from build123d import *

# Parameters (mm, degrees)
SKETCH_1_R             = 4
EXTRUDE_1_DEPTH        = 21.25
SKETCH_2_W             = 1
SKETCH_2_H             = 11
CHAMFER_1_SIZE         = 0.5
HOLE_WIZARD_M6_2_D     = 5
HOLE_WIZARD_M6_2_DEPTH = 18
HOLE_WIZARD_M6_2_TIP   = 1.502151548
HOLE_WIZARD_M4_1_D     = 3.3
HOLE_WIZARD_M4_1_DEPTH = 25
HOLE_WIZARD_M4_1_TIP   = 0.991420021
SCALE1_SCALE           = 2


with BuildPart() as part:
    # 草图1 → 凸台-拉伸1 (new, symmetric)
    with BuildSketch(Plane(origin=(0, 0, 0), x_dir=(1, 0, 0), z_dir=(0, 1, 0))):
        with Locations(Location((0, 0, 0), (0, 0, 270))):
            Circle(SKETCH_1_R)
    extrude(amount=EXTRUDE_1_DEPTH, both=True)

    # 草图2 → 旋转1 (revolve)
    with BuildSketch(Plane.XY, mode=Mode.PRIVATE) as revolve_1_sk:
        with Locations((4.5, -15.75)):
            Rectangle(SKETCH_2_W, SKETCH_2_H)
    revolve(revolve_1_sk.sketch.rotate(Axis((0, 21.25, 0), (0, -1, 0)), 270), axis=Axis((0, 21.25, 0), (0, -1, 0)))

    # 倒角1
    chamfer_1_edges = [part.edges().sort_by_distance(p)[0] for p in [
        (0, 21.25, -4),
    ]]
    chamfer(chamfer_1_edges, length=CHAMFER_1_SIZE)

    # M6 螺纹孔2
    with Locations(Plane(origin=(0, -21.25, 0), x_dir=(-1, 0, 0), z_dir=(0, -1, 0))):
        with Locations((0, 0)):
            Hole(HOLE_WIZARD_M6_2_D / 2, depth=HOLE_WIZARD_M6_2_DEPTH)
            with Locations((0, 0, -(HOLE_WIZARD_M6_2_DEPTH + HOLE_WIZARD_M6_2_TIP / 2))):  # 118° drill point
                Cone(0, HOLE_WIZARD_M6_2_D / 2, HOLE_WIZARD_M6_2_TIP, mode=Mode.SUBTRACT)

    # M4 螺纹孔1
    with Locations(Plane(origin=(0, 21.25, 0), x_dir=(1, 0, 0), z_dir=(0, 1, 0))):
        with Locations((0, 0)):
            Hole(HOLE_WIZARD_M4_1_D / 2, depth=HOLE_WIZARD_M4_1_DEPTH)
            with Locations((0, 0, -(HOLE_WIZARD_M4_1_DEPTH + HOLE_WIZARD_M4_1_TIP / 2))):  # 118° drill point
                Cone(0, HOLE_WIZARD_M4_1_D / 2, HOLE_WIZARD_M4_1_TIP, mode=Mode.SUBTRACT)


with BuildPart() as part_1:
    # Scale1: scaled about (0, -1.336200342, 0)
    add(part.part.scale(SCALE1_SCALE).moved(Location((0, 1.336200342, 0))))


solid = part_1.part
Input: part model. Units: mm. Frame: model coordinates. A direction names the side the tool comes from. Coordinates: 2 decimals unless noted, no trailing zeros. Loops run counter-clockwise (first coordinate to the right, second up) from the corner with the lowest first, then second, coordinate; pieces in that order, holes last. Notation, with made-up numbers: (80, -23) -> (134, -23) arc R33 ccw to (134, 8) -> close; hole circle Ø2 at (-32.75, 0.25). An arc over 180 degrees is marked (long way). Write item = value, one per line. Start each with the question number.
Item 1: Material intervals for line 1 (Z direction, x = -6.25, y = -16); line 2 (X direction, y = -35.5, z = 4.5); line 3 (Y direction, x = -8.25, z = 1.25), sorted ascending.
Item 2: Cut plane C-C, the plane y = 37.5. Return loops of the section in (x, z).
Item 3: Cut plane A-A, the plane z = 0. Return loops of the section in (x, y).
Item 4: First-contact query: P1, Ø3, axis at y = 22.5, z = -3, coming from the +X side; P2, Ø1, axis at y = -17, z = -6, coming from the -X side; P3, Ø1.5, axis at x = -2, y = -13, coming from the -Z side. Flat tips, straight axial feed; report the tip coordinate or a pass-through.
Item 5: Reachability of faces 1 (the face through (8.2, -19.164, 0)), 2 (the face through (2.43, 19.51, -2.23)), 3 (the face through (-1.08, -22.91, 4.88)) from +Z, -Z, +X, -X, +Y, -Y: full face, straight path, thin tool, end or side. Return the list, or none.
Item 6: Cut plane B-B, the plane x = 0. Return loops of the section in (y, z).
Item 7: Cut plane D-D, the plane y = -15. Return loops of the section in (x, z), plus the area to 3 significant figures.
Ans:
q1.line_1 = -4.99 to 4.99
q1.line_2 = -8.93 to -2.18, 2.18 to 8.93
q1.line_3 = -41.16 to -19.16
q2.outline = circle Ø16 at (0, 0); hole circle Ø6.6 at (0, 0)
q3.outline = (-10, -41.16) -> (-5, -41.16) -> (-5, -5.16) -> (-3.3, -4.14) -> (-3.3, 43.84) -> (-7, 43.84) -> (-8, 42.84) -> (-8, -19.16) -> (-10, -19.16) -> close; (3.3, -4.14) -> (5, -5.16) -> (5, -41.16) -> (10, -41.16) -> (10, -19.16) -> (8, -19.16) -> (8, 42.84) -> (7, 43.84) -> (3.3, 43.84) -> close
q4.P1 = 7.86
q4.P2 = -5.81
q4.P3 = -7.9
q5.face_1 = +Y
q5.face_2 = +Y, -Y
q5.face_3 = -Y
q6.outline = (-41.16, -10) -> (-19.16, -10) -> (-19.16, -8) -> (42.84, -8) -> (43.84, -7) -> (43.84, -3.3) -> (-4.14, -3.3) -> (-5.16, -5) -> (-41.16, -5) -> close; (-41.16, 5) -> (-5.16, 5) -> (-4.14, 3.3) -> (43.84, 3.3) -> (43.84, 7) -> (42.84, 8) -> (-19.16, 8) -> (-19.16, 10) -> (-41.16, 10) -> close
q7.outline = circle Ø16 at (0, 0); hole circle Ø10 at (0, 0)
q7.area = 123 mm²
